Input: part model. Units: mm. Frame: model coordinates. Face numbers are marked on the shaded views. Coordinates: 2 decimals unless noted, no trailing zeros. Loops run counter-clockwise (first coordinate to the right, second up) from the corner with the lowest first, then second, coordinate; pieces in that order, holes last. Notation, with made-up numbers: (34, -3.75) - (81, -3.75) arc R6 cw to (81, 7.25) - close; hole circle Ø6 at (-35, -5.5). An arc over 180 degrees is marked (long way). Use one line per item in the form item = value.
from build123d import *

# Parameters (mm, degrees)
BASENUTSKE_R  = 1.5
BASENUT_DEPTH = 1.8


with BuildPart() as part:
    # BaseNutSke → BaseNut (new body)
    with BuildSketch(Plane.XY):
        Polygon((2.75, 1.58771324), (2.75, -1.58771324), (0, -3.175426481), (-2.75, -1.58771324), (-2.75, 1.58771324), (0, 3.175426481), align=None)
        Circle(BASENUTSKE_R, mode=Mode.SUBTRACT)
    extrude(amount=-BASENUT_DEPTH)

    # Sketch3 → Double-Chamfer (revolve, cut)
    with BuildSketch(Plane(origin=(0, 0, 0), x_dir=(0, 0, -1), z_dir=(1, 0, 0))):
        Polygon((1.8, 2.75), (1.554379907, 3.175426481), (1.554379907, 13.175426481), (11.8, 13.175426481), (11.8, 2.75), align=None)
        Polygon((0.245620093, 13.175426481), (-10, 13.175426481), (-10, 2.75), (0, 2.75), (0.245620093, 3.175426481), align=None)
    revolve(axis=Axis((0, 0, 0), (0, 0, -1)), mode=Mode.SUBTRACT)

    # Sketch5 → EndChamfer (revolve, cut)
    with BuildSketch(Plane(origin=(0, 0, 0), x_dir=(0, 0, -1), z_dir=(1, 0, 0)), mode=Mode.PRIVATE) as endchamfer_sk:
        Polygon((0, 1.901666627), (0.28125, 1.5), (0, 1.5), align=None)
        Polygon((1.8, 1.901666627), (1.8, 1.5), (1.51875, 1.5), align=None)
    revolve(endchamfer_sk.sketch.rotate(Axis((0, 0, 0), (0, 0, -1)), 90), axis=Axis((0, 0, 0), (0, 0, -1)), mode=Mode.SUBTRACT)


solid = part.part
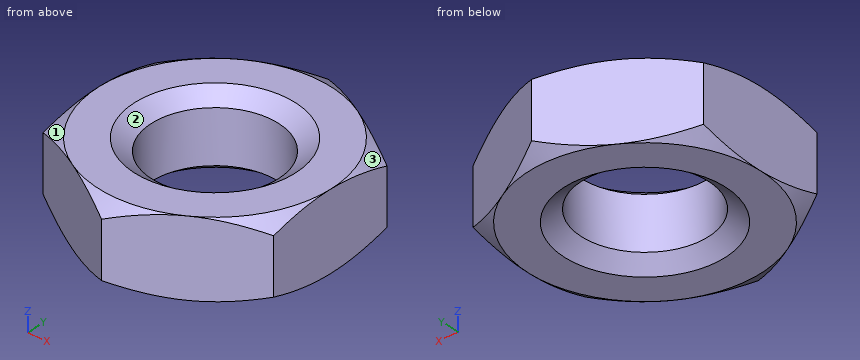
Q1. Cut plane A-A, the plane z = -1.25. Return loops of the section in (x, y), then the cut area to 3 significant figures.
Check values:
outline = (-2.75, -1.59) - (0, -3.18) - (2.75, -1.59) - (2.75, 1.59) - (0, 3.18) - (-2.75, 1.59) - close; hole circle Ø3 at (0, 0)
area = 19.1 mm²
Q2. Ray query, line 1 along Y through (x, z) = (-0.65, -0.4); line 2 along Y through (x, z) = (1.3, -0.2); line 3 along X through (y, z) = (-1.25, -0.4). Return the intervals inside material, ascending. Write a range as [from, to].
Check values:
line_1 = [-2.8, -1.35], [1.35, 2.8]
line_2 = [-2.42, -0.96], [0.96, 2.42]
line_3 = [-2.75, -0.83], [0.83, 2.75]
Q3. First-contact query: P1, Ø2, axis at x = 1, y = -1.5, coming from the +Z side. Flat tip, straight axial feed; report the tip coordinate or a pass-through.
Check values:
P1 = 0
Q4. Pull-direction query (X, two-part tool) for the marked faces 1, 2 and 3; classes: pulls with the +X half, pulls with the -X half, needs draft (parallel to the pull), parting line crosses it, or undercut.
Check values:
face_1 = pulls with the -X half
face_2 = undercut
face_3 = pulls with the +X half
